Verification items for this drawing (mm, ordinates from the low corner). A direction names the side the tool comes from. Round coordinates to 2 decimals unless told otherwise and drop trailing zeros. Order: outer loops, then holes, each group sorted by start corner. A loop starts at its lowest first (then second) coordinate and runs counter-clockwise, first axis right, second up. Notation, with made-up numbers: M 20,21.5 L 38,21.5 A16 cw 38,41.5 Z; hole C 79,6 d4. An arc over 180 degrees is marked long. One line per item, written item: value. Start each with the question number.
(1) Thickness scan on L1, parallel to X at y = 3, z = 21.2; L2, parallel to Z at x = 27, y = 5; L3, parallel to Y at x = 19, z = 12. Record the ranges inside material, lowest first.
(2) Cross-section at B-B, the plane x = 7. Enter the section's corners in (y, z).
(3) Cross-section at A-A, the plane y = 28.5. Enter the section's corners in (x, z), and give its area (3 significant figures).
(4) Cross-section at C-C, the plane y = 4. Enter the section's corners in (x, z).
(5) Access from +Z, -Z, +X, -X, +Y, -Y to the whole of each face (thin tool, end or side, straight path). Record for the marked faces 4, 5, 6, 7 and 8.
(6) Cross-section at D-D, the plane z = 12. Enter the section's corners in (x, y), and give its area (3 significant figures).
(7) Depth check by flat-ended pin: pin 1 Ø12 at (x, z) = (28.5, 21.5) entering from +Y; pin 2 Ø12 at (y, z) = (22.5, 19.5) entering from -X; pin 3 Ø6 at (x, z) = (12.5, 19.5) entering from +Y. Enter the tip coordinate at first touch or a pass-through.
(8) Release check for a two-part mould opening along Z. For the marked faces 1, 2 and 3 record: released by +Z, released by -Z, zero draft, split by the parting line, or undercut.
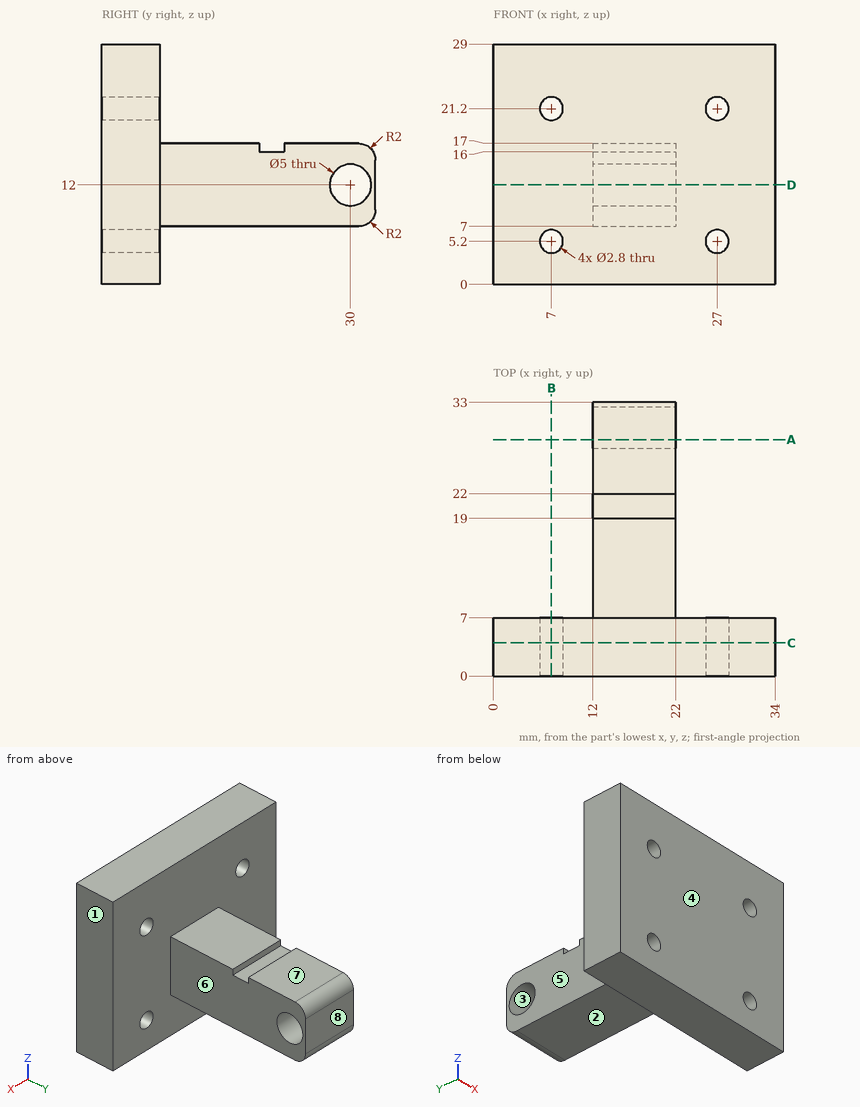
Values found:
1. L1: 0 to 5.6, 8.4 to 25.6, 28.4 to 34
1. L2: 0 to 3.8, 6.6 to 19.8, 22.6 to 29
1. L3: 0 to 27.5, 32.5 to 33
2. outline: M 0,0 L 7,0 L 7,3.8 L 0,3.8 Z; M 0,6.6 L 7,6.6 L 7,19.8 L 0,19.8 Z; M 0,22.6 L 7,22.6 L 7,29 L 0,29 Z
3. outline: M 12,7 L 22,7 L 22,10 L 12,10 Z; M 12,14 L 22,14 L 22,17 L 12,17 Z
3. area: 60.0 mm^2
4. outline: M 0,0 L 34,0 L 34,29 L 0,29 Z; hole C 7,5.2 d2.8; hole C 7,21.2 d2.8; hole C 27,5.2 d2.8; hole C 27,21.2 d2.8
5. face 4: +Z, -Z, +X, -X, -Y
5. face 5: +Z, -Z, -X, +Y
5. face 6: +Z, -Z, +X, +Y
5. face 7: +Z, +X, -X, +Y
5. face 8: +Z, -Z, +X, -X, +Y
6. outline: M 0,0 L 34,0 L 34,7 L 22,7 L 22,27.5 L 12,27.5 L 12,7 L 0,7 Z; M 12,32.5 L 22,32.5 L 22,33 L 12,33 Z
6. area: 448 mm^2
7. pin 1: y = 7
7. pin 2: x = 12
7. pin 3: y = 32.32
8. face 1: zero draft
8. face 2: released by -Z
8. face 3: undercut
